Design review of the part built by this model. Coordinates are the model's own, in mm. Coordinates: 2 decimals unless noted, no trailing zeros. Loops run counter-clockwise (first coordinate to the right, second up) from the corner with the lowest first, then second, coordinate; pieces in that order, holes last. Notation, with made-up numbers: M 65.25,-16 L 107.25,-16 A20 ccw 107.25,-2 Z; hole C 0.25,-32 d2. An arc over 180 degrees is marked long. Write item = value, one per line. Start each with the question number.
```python
from build123d import *

# Parameters (mm, degrees)
SKETCH1_R           = 2
SKETCH1_R_2         = 3.25
BOSS_EXTRUDE1_DEPTH = 7
SKETCH2_R           = 5.15
CUT_EXTRUDE1_DEPTH  = 2
CUT_EXTRUDE3_DEPTH  = 2


with BuildPart() as part:
    # Sketch1 → Boss-Extrude1 (new body)
    with BuildSketch(Plane(origin=(0, 0, 0), x_dir=(1, 0, 0), z_dir=(0, 1, 0))):
        with BuildLine():
            Line((-118.197336116, 56.752063188), (69.085931957, 56.752063188))
            ThreePointArc((69.085931957, 56.752063188), (72.621465863, 55.287597094), (74.085931957, 51.752063188))
            Line((74.085931957, 51.752063188), (74.085931957, -66.247936812))
            ThreePointArc((74.085931957, -66.247936812), (72.621465863, -69.783470718), (69.085931957, -71.247936812))
            Line((69.085931957, -71.247936812), (-118.197336116, -71.247936812))
            ThreePointArc((-118.197336116, -71.247936812), (-121.732870022, -69.783470718), (-123.197336116, -66.247936812))
            Line((-123.197336116, -66.247936812), (-123.197336116, 51.752063188))
            ThreePointArc((-123.197336116, 51.752063188), (-121.732870022, 55.287597094), (-118.197336116, 56.752063188))
        make_face()
        with Locations(Location((-118.197336116, 51.752063188, 0), (0, 0, 270))):
            Circle(SKETCH1_R, mode=Mode.SUBTRACT)
        with Locations(Location((69.085931957, -66.247936812, 0), (0, 0, 270))):
            Circle(SKETCH1_R, mode=Mode.SUBTRACT)
        with Locations(Location((44.085931957, 42.752063188, 0), (0, 0, 270))):
            Circle(SKETCH1_R, mode=Mode.SUBTRACT)
        with Locations(Location((-0.914068043, 42.752063188, 0), (0, 0, 270))):
            Circle(SKETCH1_R, mode=Mode.SUBTRACT)
        with Locations(Location((-93.197336116, -57.247936812, 0), (0, 0, 270))):
            Circle(SKETCH1_R, mode=Mode.SUBTRACT)
        with Locations(Location((-48.197336116, -57.247936812, 0), (0, 0, 270))):
            Circle(SKETCH1_R, mode=Mode.SUBTRACT)
        with Locations(Location((-76.697336116, 10.252063188, 0), (0, 0, 270))):
            Circle(SKETCH1_R_2, mode=Mode.SUBTRACT)
        with Locations(Location((27.585931957, -24.747936812, 0), (0, 0, 270))):
            Circle(SKETCH1_R_2, mode=Mode.SUBTRACT)
    extrude(amount=BOSS_EXTRUDE1_DEPTH)

    # Sketch2 → Cut-Extrude1 (cut)
    with BuildSketch(Plane.XZ):
        with Locations((-118.197336116, -51.752063188)):
            Circle(SKETCH2_R)
        with Locations(Location((-0.914068043, -42.752063188, 0), (0, 0, 270))):
            Circle(SKETCH2_R)
        with Locations(Location((44.085931957, -42.752063188, 0), (0, 0, 270))):
            Circle(SKETCH2_R)
        with Locations((69.085931957, 66.247936812)):
            Circle(SKETCH2_R)
        with Locations(Location((-48.197336116, 57.247936812, 0), (0, 0, 270))):
            Circle(SKETCH2_R)
        with Locations(Location((-93.197336116, 57.247936812, 0), (0, 0, 270))):
            Circle(SKETCH2_R)
    extrude(amount=-CUT_EXTRUDE1_DEPTH, mode=Mode.SUBTRACT)

    # Sketch4 → Cut-Extrude3 (cut)
    with BuildSketch(Plane(origin=(0, 7, 0), x_dir=(1, 0, 0), z_dir=(0, 1, 0))):
        with BuildLine():
            ThreePointArc((-16.825362278, -7.247936812), (-22.411093503, 0.178960757), (-31.096095238, -3.127086078))
            Line((-31.096095238, -3.127086078), (-28.557891229, -4.726311018))
            ThreePointArc((-28.557891229, -4.726311018), (-23.243375898, -2.703279), (-19.825362278, -7.247936812))
            ThreePointArc((-19.825362278, -7.247936812), (-20.011044267, -8.560262993), (-20.553512929, -9.769562607))
            Line((-20.553512929, -9.769562607), (-18.01530892, -11.368787546))
            ThreePointArc((-18.01530892, -11.368787546), (-17.12880451, -9.392545389), (-16.825362278, -7.247936812))
        make_face()
        with BuildLine():
            Line((-28.557891229, -4.726311018), (-31.096095238, -3.127086078))
            ThreePointArc((-31.096095238, -3.127086078), (-28.676552813, -13.788329971), (-18.01530892, -11.368787546))
            Line((-18.01530892, -11.368787546), (-20.553512929, -9.769562607))
            ThreePointArc((-20.553512929, -9.769562607), (-27.077327874, -11.250125962), (-28.557891229, -4.726311018))
        make_face()
        with BuildLine():
            ThreePointArc((-1.038546315, -7.247936812), (-15.286948513, 35.660240122), (-52.943648692, 10.638218929))
            Line((-52.943648692, 10.638218929), (-50.005532279, 8.78702453))
            ThreePointArc((-50.005532279, 8.78702453), (-17.529440865, 33.223292942), (-2.972559683, -4.723049934))
            ThreePointArc((-2.972559683, -4.723049934), (-19.617614772, 4.759547304), (-38.501589456, 1.538831635))
            Line((-38.501589456, 1.538831635), (-35.563473042, -0.312362764))
            ThreePointArc((-35.563473042, -0.312362764), (-18.963238247, 1.569321693), (-4.772942827, -7.247936812))
            ThreePointArc((-4.772942827, -7.247936812), (-8.774709253, -11.203752107), (-13.547931116, -14.18351086))
            Line((-13.547931116, -14.18351086), (-10.609814702, -16.034705259))
            ThreePointArc((-10.609814702, -16.034705259), (-6.517387874, -13.237701677), (-2.972559683, -9.77282369))
            ThreePointArc((-2.972559683, -9.77282369), (-0.088261351, -16.255690409), (0.89412812, -23.282898154))
            Line((0.89412812, -23.282898154), (3.832244534, -25.134092553))
            ThreePointArc((3.832244534, -25.134092553), (2.894499286, -15.78317183), (-1.038546315, -7.247936812))
        make_face()
        with BuildLine():
            Line((-50.005532279, 8.78702453), (-52.943648692, 10.638218929))
            ThreePointArc((-52.943648692, 10.638218929), (-52.005903444, 1.287298206), (-48.072857843, -7.247936812))
            ThreePointArc((-48.072857843, -7.247936812), (-33.824455645, -50.156113746), (3.832244534, -25.134092553))
            Line((3.832244534, -25.134092553), (0.89412812, -23.282898154))
            ThreePointArc((0.89412812, -23.282898154), (-31.581963293, -47.719166566), (-46.138844475, -9.77282369))
            ThreePointArc((-46.138844475, -9.77282369), (-29.493789386, -19.255420928), (-10.609814702, -16.034705259))
            Line((-10.609814702, -16.034705259), (-13.547931116, -14.18351086))
            ThreePointArc((-13.547931116, -14.18351086), (-30.148165911, -16.065195317), (-44.338461331, -7.247936812))
            ThreePointArc((-44.338461331, -7.247936812), (-40.336694905, -3.292121517), (-35.563473042, -0.312362764))
            Line((-35.563473042, -0.312362764), (-38.501589456, 1.538831635))
            ThreePointArc((-38.501589456, 1.538831635), (-42.594016284, -1.258171947), (-46.138844475, -4.723049934))
            ThreePointArc((-46.138844475, -4.723049934), (-49.023142808, 1.759816785), (-50.005532279, 8.78702453))
        make_face()
    extrude(amount=-CUT_EXTRUDE3_DEPTH, mode=Mode.SUBTRACT)


solid = part.part
```
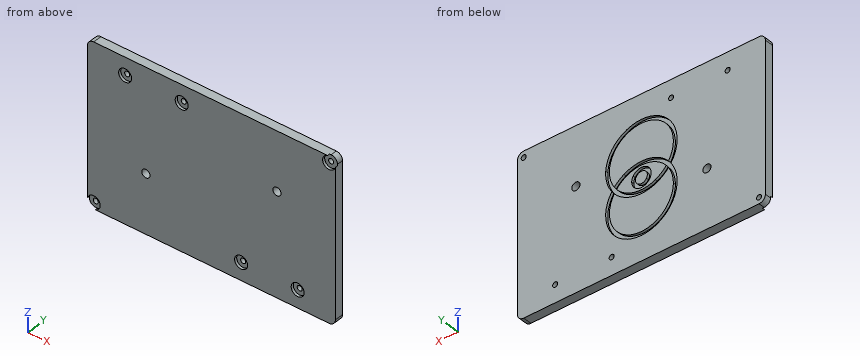
(1) Insertion check: pin 1 (3 mm diameter, centred on x = -1, z = -44, fed in from -Y). The pin has a flat end and moves straight along its axis. Give the tip position at first contact, or say it passes through.
(2) Take a section at A-A (z = -31.5). State the section outline as (x, y) points.
(3) To check wall thickness, follow L1, parallel to X at y = 5.75, z = -5.5; L2, parallel to Z at x = -76.5, y = 6; L3, parallel to X at y = 0.5, z = -10. State the ranges of each line that lie inside material, in increasing order.
Results list:
q1.pin_1 = 2
q2.outline = M -123.2,0 L 74.09,0 L 74.09,7 L -7.46,7 L -7.46,5 L -13.12,5 L -13.12,7 L -35.99,7 L -35.99,5 L -41.66,5 L -41.66,7 L -123.2,7 Z
q3.L1 = -123.2 to -52.82, -49.8 to 0.68, 3.71 to 74.09
q3.L2 = -56.75 to -13.5, -7.01 to 71.25
q3.L3 = -123.2 to -79.94, -73.46 to 74.09
